Autodesk Inventor part; units mm, degrees
ref_plane "YZ Plane" through (0, 0, 0) normal (1, 0, 0) x (0, 1, 0)
ref_plane "XZ Plane" through (0, 0, 0) normal (0, 1, 0) x (-1, 0, 0)
ref_plane "XY Plane" through (0, 0, 0) normal (0, 0, 1) x (1, 0, 0)
sketch "Sketch1" plane through (0, 0, 0) normal (1, 0, 0) x (0, 1, 0)
  line L0 (3.5, -7) -> (-3.5, -7)
  line L1 (-3.5, -7) -> (-3.5, 7)
  line L2 (-3.5, 7) -> (3.5, 7)
  line L3 (3.5, 7) -> (3.5, -7)
  line L4 (3.5, -7) -> (-3.5, 7) construction
  line L5 (-3.5, -7) -> (3.5, 7) construction
  point P0 (0, 0)
  dimension "d0" = 7
  dimension "d1" = 14
extrude "Extrusion1" add sketch "Sketch1" along normal blind 152.4 and the other way blind 50.8
sketch "Sketch2" plane through (-50.8, 3.5, 7) normal (0, 1, 0) x (1, 0, 0)
  circle A0 centre (56.8, 7) radius 2
  point P0 (50.8, 7)
  dimension "d4" = 4
  dimension "d5" = 6
extrude "Extrusion2" cut sketch "Sketch2" against normal through all
sketch "Sketch3" plane through (-50.8, 3.5, 7) normal (0, 1, 0) x (1, 0, 0)
  line L0 (203.2, 0) -> (193.2, 0)
  line L1 (193.2, 0) -> (193.2, 14)
  line L2 (193.2, 14) -> (203.2, 14)
  line L3 (203.2, 14) -> (203.2, 0)
  line L4 (203.2, 0) -> (0, 0)
  line L5 (203.2, 14) -> (203.2, 0)
  point P0 (50.8, 7)
  dimension "d8" = 10
  dimension "d9" = 14
  dimension "d10" = 0
  dimension "d11" = 0
extrude "Extrusion3" add sketch "Sketch3" along normal blind 100
sketch "Sketch5" plane through (142.4, 3.5, -7) normal (-1, 0, 0) x (0, 0, 1)
  line L0 (14, 100) -> (0, 100)
  line L1 (0, 100) -> (0, 93)
  line L2 (0, 93) -> (14, 93)
  line L3 (14, 93) -> (14, 100)
  line L4 (14, 0) -> (14, 100)
  line L5 (0, 100) -> (14, 100)
  point P0 (7, -3.5)
  dimension "d17" = 14
  dimension "d18" = 7
  dimension "d19" = 0
  dimension "d20" = 0
extrude "Extrusion4" add sketch "Sketch5" along normal blind 25
sketch "Sketch10" plane through (-50.8, 3.5, 7) normal (0, 1, 0) x (1, 0, 0)
  point P0 (50.8, 7)
sketch "Sketch11" plane through (-50.8, 0, 0) normal (-1, 0, 0) x (0, 0, 1)
  point P0 (0, 0)
sketch "Sketch12" plane through (152.4, 0, 0) normal (1, 0, 0) x (0, 0, -1)
  point P0 (0, 0)
sketch "Sketch13" plane through (-50.8, 103.5, 7) normal (0, 1, 0) x (1, 0, 0)
  point P0 (50.8, 7)
properties part number "handle" material "PBT Plastic"
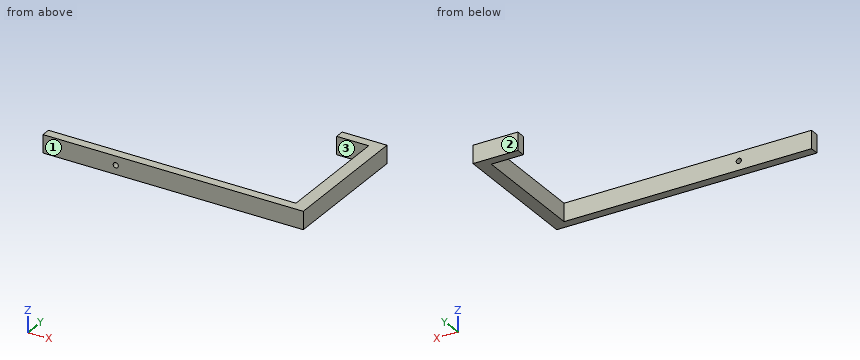
Could you check a few things on this model? Use its own coordinates, in mm. Face numbers are marked on the shaded views. Round coordinates to 2 decimals unless told otherwise and drop trailing zeros. Loops run counter-clockwise (first coordinate to the right, second up) from the corner with the lowest first, then second, coordinate; pieces in that order, holes last. Notation, with made-up numbers: (5.5, 54.25) -> (48.5, 54.25) arc R11 ccw to (48.5, 65.25) -> close; hole circle Ø5 at (37, -6). An arc over 180 degrees is marked (long way). Use CSV: the item, a comma, the result in double quotes.
(1) Suppose I cut it at B-B on z = 0. Write out the boundary of the cut face in (x, y).
Return value:
outline,"(-50.8, -3.5) -> (4, -3.5) -> (4, 3.5) -> (-50.8, 3.5) -> close; (8, -3.5) -> (152.4, -3.5) -> (152.4, 103.5) -> (117.4, 103.5) -> (117.4, 96.5) -> (142.4, 96.5) -> (142.4, 3.5) -> (8, 3.5) -> close"
(2) Suppose I cut it at A-A on x = 6. Write out the boundary of the cut face in (y, z), plus the area to 3 significant figures.
Return value:
outline,"(-3.5, -7) -> (3.5, -7) -> (3.5, -2) -> (-3.5, -2) -> close; (-3.5, 2) -> (3.5, 2) -> (3.5, 7) -> (-3.5, 7) -> close"
area,"70.0 mm²"
(3) Will these pins go through, and if not, where does the flat tip stop? pin 1 Ø6 at (x, z) = (98.5, 0.5) entering from +Y; pin 2 Ø2 at (y, z) = (86, 5) entering from -X; pin 3 Ø3.5 at (y, z) = (99.5, 1) entering from -X.
Return value:
pin 1,"stops at y = 3.5"
pin 2,"stops at x = 142.4"
pin 3,"stops at x = 117.4"
(4) Suppose I cut it at C-C on y = 31. Write out the boundary of the cut face in (x, z), plus the area to 3 significant figures.
Return value:
outline,"(142.4, -7) -> (152.4, -7) -> (152.4, 7) -> (142.4, 7) -> close"
area,"140 mm²"
(5) If we mould it in two halves opening along Y, with no side actions, what happens to the marked faces 1, 2 and 3? For each: +Y half, -Y half, draft (parallel to the pull), parting line (faces both ways), or undercut.
Return value:
face 1,"-Y half"
face 2,"+Y half"
face 3,"undercut"
(6) If I drill on probe 1 along Z at (x, y) = (6, 0); probe 2 along Y at (x, z) = (140.5, 5.75); probe 3 along X at (y, z) = (85, 2.75), over which ranges is the centre line in solid material (lowest first)? Write a range as [from, to].
Return value:
probe 1,"z = [-7, -2], [2, 7]"
probe 2,"y = [-3.5, 3.5], [96.5, 103.5]"
probe 3,"x = [142.4, 152.4]"
